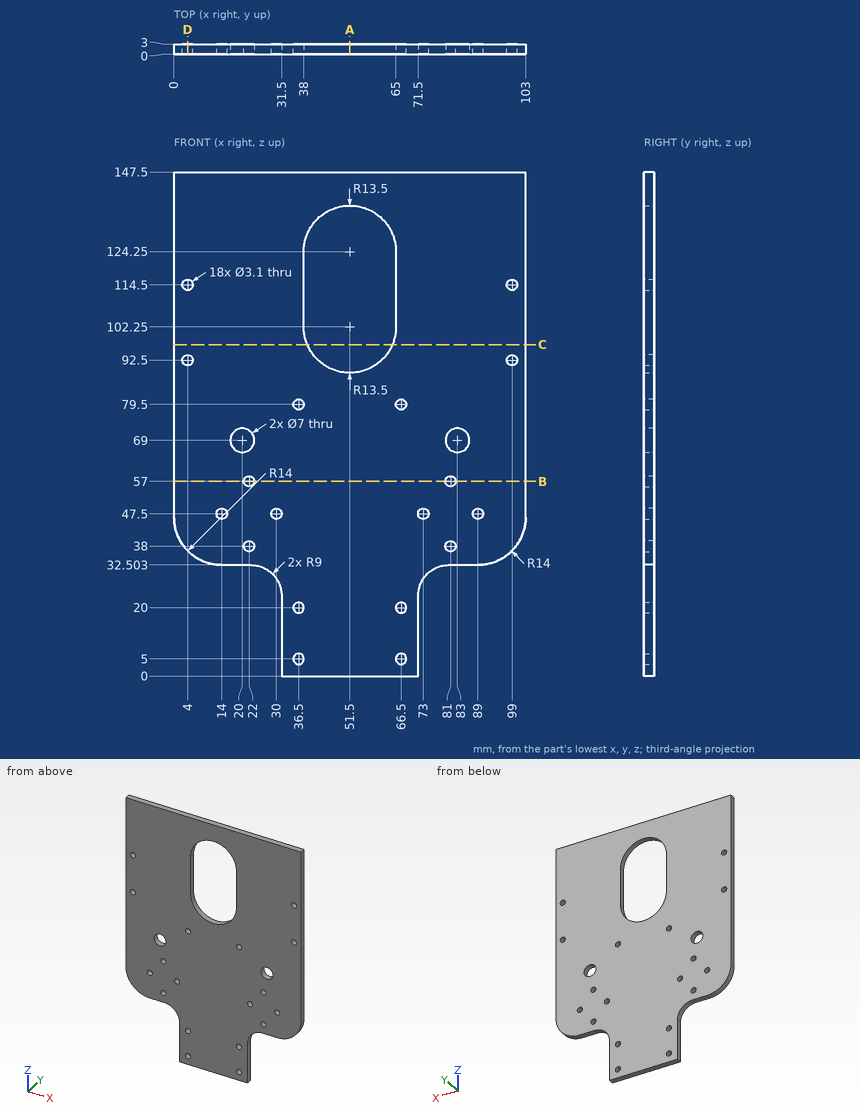
Job drawing, mm, ordinate dimensions from the low corner. One solid piece. Give positions to 0.01 mm unless a question says otherwise; leave off trailing zeros. Loops run counter-clockwise (first coordinate to the right, second up) from the corner with the lowest first, then second, coordinate; pieces in that order, holes last. Notation, with made-up numbers: (82, 31) -> (88, 31) arc R15 cw to (88, 51) -> close; hole circle Ø5 at (13.5, -32.75). An arc over 180 degrees is marked (long way). Write each question's results on one line, items separated by ' | '.
(1) Flat gauge pins, fed straight in: pin 1 Ø0.9 at (x, y) = (17, 2) entering from -Z; pin 2 Ø1.5 at (y, z) = (1, 8) entering from +X; pin 3 Ø1.5 at (y, z) = (2, 14) entering from -X. Where does each tip first touch, or does it go through?
Geometry results:
pin 1: stops at z = 32.5 | pin 2: stops at x = 71.5 | pin 3: stops at x = 31.5
(2) Probe line 1 along X through (y, z) = (0.8, 69); line 2 along X through (y, z) = (1.45, 5); line 3 along X through (y, z) = (1.7, 47.5). List the from-to ranges inside material, lowest first.
Geometry results:
line 1: x = 0 to 16.5, 23.5 to 79.5, 86.5 to 103 | line 2: x = 31.5 to 34.95, 38.05 to 64.95, 68.05 to 71.5 | line 3: x = 0 to 12.45, 15.55 to 28.45, 31.55 to 71.45, 74.55 to 87.45, 90.55 to 103
(3) Cut at B-B on z = 57. List the corners of the cut face in (x, y).
Geometry results:
outline: (0, 0) -> (20.45, 0) -> (20.45, 3) -> (0, 3) -> close; (23.55, 0) -> (79.45, 0) -> (79.45, 3) -> (23.55, 3) -> close; (82.55, 0) -> (103, 0) -> (103, 3) -> (82.55, 3) -> close
(4) Cut at A-A on x = 51.5. List the corners of the cut face in (y, z), and give its area (4 significant figures).
Geometry results:
outline: (0, 0) -> (3, 0) -> (3, 88.75) -> (0, 88.75) -> close; (0, 137.75) -> (3, 137.75) -> (3, 147.5) -> (0, 147.5) -> close | area: 295.5 mm²
(5) Cut at D-D on x = 4. List the corners of the cut face in (y, z), and give its area (3 significant figures).
Geometry results:
outline: (0, 36.71) -> (3, 36.71) -> (3, 90.95) -> (0, 90.95) -> close; (0, 94.05) -> (3, 94.05) -> (3, 112.95) -> (0, 112.95) -> close; (0, 116.05) -> (3, 116.05) -> (3, 147.5) -> (0, 147.5) -> close | area: 314 mm²
(6) Cut at C-C on z = 97. List the corners of the cut face in (x, y), and give its area (3 significant figures).
Geometry results:
outline: (0, 0) -> (39.06, 0) -> (39.06, 3) -> (0, 3) -> close; (63.94, 0) -> (103, 0) -> (103, 3) -> (63.94, 3) -> close | area: 234 mm²
